Verification items for the finished model (mm, model axes). Face numbers are marked on the shaded views. A direction names the side the tool comes from. Coordinates: 2 decimals unless noted, no trailing zeros. Loops run counter-clockwise (first coordinate to the right, second up) from the corner with the lowest first, then second, coordinate; pieces in that order, holes last. Notation, with made-up numbers: M -33,42 L 3,42 A15 ccw 3,46 Z; hole C -24,49.25 d8. An arc over 180 degrees is marked long. Write item = value, one per line. Start each with the question number.
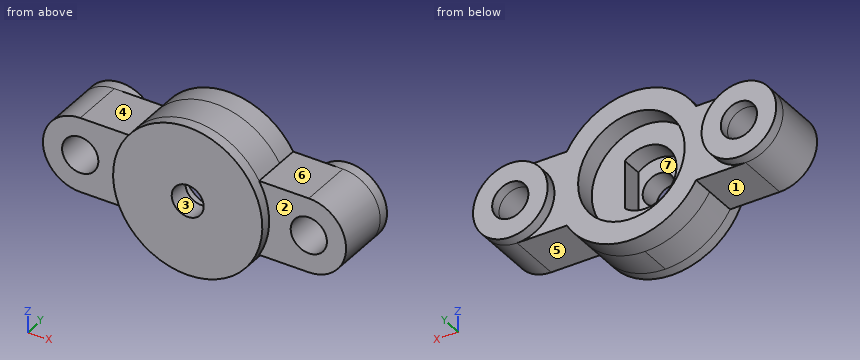
```python
from build123d import *
from build123d.topology import SkipClean

# Parameters (mm, degrees)
ESQUISSE1_R             = 5
ESQUISSE1_R_2           = 1.7
BOSS_EXTRU_1_DEPTH      = 5
ESQUISSE2_R             = 3.5
ESQUISSE2_R_2           = 1.7
BOSS_EXTRU_2_DEPTH      = 1
BOSS_EXTRU_3_DEPTH      = 1
BOSS_EXTRU_3_DEPTH_BACK = 3
ESQUISSE3_R             = 7
ESQUISSE3_R_2           = 1.5
ENL_V_MAT_EXTRU_1_DEPTH = 2


with BuildPart() as part:
    # Esquisse1 → Boss.-Extru.1 (new body)
    with BuildSketch(Plane(origin=(0, 0, 0), x_dir=(1, 0, 0), z_dir=(0, 1, 0))):
        with BuildLine():
            Line((-10.72, 3.5), (-6.062177826, 3.5))
            ThreePointArc((-6.062177826, 3.5), (0, 7), (6.062177826, 3.5))
            Line((6.062177826, 3.5), (10.72, 3.5))
            ThreePointArc((10.72, 3.5), (14.22, 0), (10.72, -3.5))
            Line((10.72, -3.5), (6.062177826, -3.5))
            ThreePointArc((6.062177826, -3.5), (0, -7), (-6.062177826, -3.5))
            Line((-6.062177826, -3.5), (-10.72, -3.5))
            ThreePointArc((-10.72, -3.5), (-14.22, 0), (-10.72, 3.5))
        make_face()
        with Locations(Location((0, 0, 0), (0, 0, 270))):
            Circle(ESQUISSE1_R, mode=Mode.SUBTRACT)
        with Locations(Location((10.72, 0, 0), (0, 0, 270))):
            Circle(ESQUISSE1_R_2, mode=Mode.SUBTRACT)
        with Locations(Location((-10.72, 0, 0), (0, 0, 270))):
            Circle(ESQUISSE1_R_2, mode=Mode.SUBTRACT)
    extrude(amount=BOSS_EXTRU_1_DEPTH)

    # Esquisse2 → Boss.-Extru.2 (add)
    # profile 1 of 2: a face of its own
    with SkipClean():  # the faces are left unmerged after this step: merging them gives an invalid solid
        with BuildSketch(Plane(origin=(0, 5, 0), x_dir=(1, 0, 0), z_dir=(0, 1, 0))):
            with Locations(Location((-10.72, 0, 0), (0, 0, 270))):
                Circle(ESQUISSE2_R)
            with Locations(Location((-10.72, 0, 0), (0, 0, 270))):
                Circle(ESQUISSE2_R_2, mode=Mode.SUBTRACT)
        # profile 2 of 2: a face of its own
        with BuildSketch(Plane(origin=(0, 5, 0), x_dir=(1, 0, 0), z_dir=(0, 1, 0))):
            with Locations(Location((10.72, 0, 0), (0, 0, 270))):
                Circle(ESQUISSE2_R)
            with Locations(Location((10.72, 0, 0), (0, 0, 270))):
                Circle(ESQUISSE2_R_2, mode=Mode.SUBTRACT)
        extrude(amount=BOSS_EXTRU_2_DEPTH)

    # Esquisse3 → Boss.-Extru.3 (add, two sides: drawn at the far end of the back side and taken through both)
    with SkipClean():  # the faces are left unmerged after this step: merging them gives an invalid solid
        with BuildSketch(Plane.XZ.offset(-BOSS_EXTRU_3_DEPTH_BACK)):
            with Locations(Location((0, 0, 0), (0, 0, 270))):
                Circle(ESQUISSE3_R)
            with Locations(Location((0, 0, 0), (0, 0, 270))):
                Circle(ESQUISSE3_R_2, mode=Mode.SUBTRACT)
        extrude(amount=BOSS_EXTRU_3_DEPTH + BOSS_EXTRU_3_DEPTH_BACK)

    # Esquisse6 → Enl_v. mat.-Extru.1 (cut)
    with SkipClean():  # the faces are left unmerged after this step: merging them gives an invalid solid
        with BuildSketch(Plane(origin=(0, 3, 0), x_dir=(1, 0, 0), z_dir=(0, 1, 0))):
            with BuildLine():
                Line((1.9, 2.256656819), (1.9, -2.256656819))
                ThreePointArc((1.9, -2.256656819), (-2.95, 0), (1.9, 2.256656819))
            make_face()
        extrude(amount=-ENL_V_MAT_EXTRU_1_DEPTH, mode=Mode.SUBTRACT)


solid = part.part
```
Q1. Gauge pin test, flat ends, axial feed: pin 1 (1.4 mm diameter, centred on x = 8.5, y = 2, fed in from +Z); pin 2 (5.5 mm diameter, centred on x = 10.72, z = 0, fed in from +Y); pin 3 (2 mm diameter, centred on x = 6.5, y = 0, fed in from +Z); pin 4 (2 mm diameter, centred on x = 8.5, z = 0.5, fed in from -Y). Record the tip position at first contact, or that the pin passes through.
Q2. Set-up check for the marked faces 4, 5, 6 and 7: record each of +Z, -Z, +X, -X, +Y, -Y from which the full face is reachable in a straight line by a thin tool's end or side.
Q3. Sectioned sample at B-B on z = 0. Count the separate pieces of the cut face and the enclosed holes in it, plus the area to 3 significant figures.
Q4. Sectioned sample at D-D on y = 2.5. Record the cut outline in (x, z), plus the area to 3 significant figures.
Q5. Mould release check, pull along Z, two halves, no side actions. Record for the marked faces 1, 2 and 3: +Z half, -Z half, draft (parallel to the pull), parting line (faces both ways), or undercut.
Q6. Scan lines: L1, parallel to X at y = 5.7, z = 0; L2, parallel to X at y = 1.4, z = 0; L3, parallel to Y at x = -2.25, z = -5. Record each from-to range of solid material in increasing order. Write a range as [from, to].
Q7. Sectioned sample at A-A on y = 0.5. Record the cut outline in (x, z).
Q8. Sectioned sample at C-C on x = 8.5. Record the cut outline in (y, z), plus the area to 3 significant figures.
Solutions:
q1.pin_1 = 3.5
q1.pin_2 = 6
q1.pin_3 = 4.33
q1.pin_4 = 0
q2.face_4 = +Z, -X, +Y, -Y
q2.face_5 = -Z, +X, +Y, -Y
q2.face_6 = +Z, +X, +Y, -Y
q2.face_7 = +Y
q3.separate_pieces = 4
q3.enclosed_holes = 0
q3.area = 93.7 mm²
q4.outline = M -10.72,-3.5 L -6.06,-3.5 A7 ccw 6.06,-3.5 L 10.72,-3.5 A3.5 ccw 10.72,3.5 L 6.06,3.5 A7 ccw -6.06,3.5 L -10.72,3.5 A3.5 ccw Z; hole C -10.72,0 d3.4; hole M 1.9,-2.26 L 1.9,2.26 A2.95 ccw long Z; hole C 10.72,0 d3.4
q4.area = 207 mm²
q5.face_1 = -Z half
q5.face_2 = draft
q5.face_3 = undercut
q6.L1 = [-14.22, -12.42], [-9.02, -7.22], [7.22, 9.02], [12.42, 14.22]
q6.L2 = [-14.22, -12.42], [-9.02, -2.95], [1.9, 9.02], [12.42, 14.22]
q6.L3 = [-1, 5]
q7.outline = M -10.72,-3.5 L -6.06,-3.5 A7 ccw 6.06,-3.5 L 10.72,-3.5 A3.5 ccw 10.72,3.5 L 6.06,3.5 A7 ccw -6.06,3.5 L -10.72,3.5 A3.5 ccw Z; hole C -10.72,0 d3.4; hole C 0,0 d3; hole C 10.72,0 d3.4
q8.outline = M 0,-3.5 L 5,-3.5 L 5,-2.71 L 6,-2.71 L 6,2.71 L 5,2.71 L 5,3.5 L 0,3.5 Z
q8.area = 40.4 mm²
